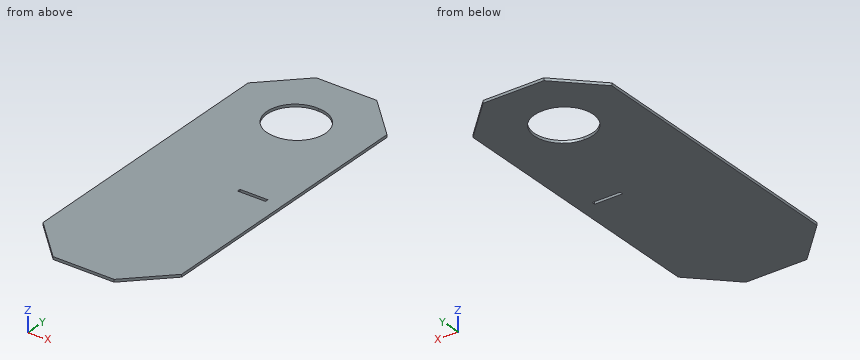
from build123d import *

# Parameters (mm, degrees)
EXTRUDE_1_DEPTH     = 4
CUT_EXTRUDE_1_DEPTH = 650.396885451
SKETCH_3_W          = 42.169531332
SKETCH_3_H          = 5.000000403
CUT_EXTRUDE_2_DEPTH = 650.396885451


with BuildPart() as part:
    # Эскиз1 → Вытянуть1 (new body)
    with BuildSketch(Plane.XY):
        Polygon((105.082921559, 581.722068254), (45.979042749, 640.825947064), (-45.813199631, 640.825947064), (-104.917078441, 581.722068254), (-104.917078441, 162.212880509), (-45.97317451, 103.268976578), (46.326817337, 103.268976578), (105.082921559, 162.0250808), align=None)
    extrude(amount=EXTRUDE_1_DEPTH)

    # Эскиз2 → Вырез-Вытянуть1 (cut, through all)
    with BuildSketch(Plane.XY.offset(4)):
        with BuildLine():
            ThreePointArc((0.117260776, 497.024602251), (43.117260776, 540.024602251), (0.117260776, 583.024602251))
            ThreePointArc((0.117260776, 583.024602251), (-45.765193681, 540.024602251), (0.117260776, 497.024602251))
        make_face()
    extrude(amount=-CUT_EXTRUDE_1_DEPTH, mode=Mode.SUBTRACT)

    # Эскиз3 → Вырез-Вытянуть2 (cut, through all)
    with BuildSketch(Plane(origin=(0, 0, 0), x_dir=(-1, 0, 0), z_dir=(0, 0, -1))):
        with Locations((-61.103979415, 366.588061036)):
            Rectangle(SKETCH_3_W, SKETCH_3_H)
    extrude(amount=-CUT_EXTRUDE_2_DEPTH, mode=Mode.SUBTRACT)


solid = part.part
Read the model definition and answer for the solid it produces. Units are mm, in the model's axes. Coordinates: 2 decimals unless noted, no trailing zeros. Write each loop counter-clockwise with the first axis right and the second up, starting at its lowest first coordinate (ties: lowest second). Pieces come first, ordered by that corner, then holes. Notation, with made-up numbers: (83.25, -13) - (87.25, -13) arc R17 ccw to (87.25, 14) - close; hole circle Ø10 at (44.25, 88). An arc over 180 degrees is marked (long way). One line per question, with ' | ' between items.
Q1. Consider L1, parallel to Y at x = 0, z = 1; L2, parallel to Y at x = -38, z = 2; L3, parallel to X at y = 575, z = 2.25. Determine where each line is inside the solid, lowest interval first. Write a range as [from, to].
Result set:
L1: [103.27, 497.02], [583.03, 640.83] | L2: [103.27, 515.35], [564.7, 640.83] | L3: [-104.92, -27.84], [25.13, 105.08]
Q2. Find section A-A, the plane z = 2.65. Write down the section's boundary in (x, y), plus the area to 3 significant figures.
Result set:
outline: (-104.92, 162.21) - (-45.97, 103.27) - (46.33, 103.27) - (105.08, 162.03) - (105.08, 581.72) - (45.98, 640.83) - (-45.81, 640.83) - (-104.92, 581.72) - close; hole (0.12, 497.02) arc R43 ccw to (0.12, 583.02) arc R43.09 ccw (long way) to start; hole (40.02, 364.09) - (82.19, 364.09) - (82.19, 369.09) - (40.02, 369.09) - close | area: 99,700 mm^2
Q3. Each of these flat-tipped pins is pushed along its axis until it touches: P1, Ø1.5, axis at x = 28.5, y = 326.5, coming from the -Z side; P2, Ø1.2, axis at x = 51, z = 1.5, coming from the -Y side; P3, Ø2, axis at x = 58.5, z = 1, coming from the +Y side (3 decimals). Where does it stop, or does it pass through?
Result set:
P1: z = 0 | P2: y = 107.34 | P3: y = 629.305
Q4. Find section C-C, the plane x = 74. Write down the section's boundary in (y, z).
Result set:
outline: (130.94, 0) - (364.09, 0) - (364.09, 4) - (130.94, 4) - close; (369.09, 0) - (612.8, 0) - (612.8, 4) - (369.09, 4) - close
Q5. Find section B-B, the plane x = 53. Write down the section's boundary in (y, z).
Result set:
outline: (109.94, 0) - (364.09, 0) - (364.09, 4) - (109.94, 4) - close; (369.09, 0) - (633.8, 0) - (633.8, 4) - (369.09, 4) - close
